```python
from build123d import *

# Parameters (mm, degrees)
SKETCH2_R           = 15.875
SKETCH2_R_2         = 2.54
BOSS_EXTRUDE1_DEPTH = 3.175
FILLET1_R           = 2.54


with BuildPart() as part:
    # Sketch2 → Boss-Extrude1 (new body)
    with BuildSketch(Plane.XY):
        Polygon((-508, 25.4), (-481.624580264, 25.4), (-457.99375, 25.4), (-431.8, 25.4), (-368.3, 25.4), (-368.3, -25.4), (-431.8, -25.4), (-457.99375, -25.4), (-481.624580264, -25.4), (-508, -25.4), align=None)
        with Locations((-469.9, 0)):
            Circle(SKETCH2_R, mode=Mode.SUBTRACT)
        with Locations((-495.3, 12.7)):
            Circle(SKETCH2_R_2, mode=Mode.SUBTRACT)
        with Locations((-495.3, -12.7)):
            Circle(SKETCH2_R_2, mode=Mode.SUBTRACT)
        with Locations((-444.5, -12.7)):
            Circle(SKETCH2_R_2, mode=Mode.SUBTRACT)
        with Locations((-431.8, -12.7)):
            Circle(SKETCH2_R_2, mode=Mode.SUBTRACT)
        with Locations((-419.1, -12.7)):
            Circle(SKETCH2_R_2, mode=Mode.SUBTRACT)
        with Locations((-419.1, 0)):
            Circle(SKETCH2_R_2, mode=Mode.SUBTRACT)
        with Locations((-431.8, 0)):
            Circle(SKETCH2_R_2, mode=Mode.SUBTRACT)
        with Locations((-431.8, 12.7)):
            Circle(SKETCH2_R_2, mode=Mode.SUBTRACT)
        with Locations((-419.1, 12.7)):
            Circle(SKETCH2_R_2, mode=Mode.SUBTRACT)
        with Locations((-444.5, 12.7)):
            Circle(SKETCH2_R_2, mode=Mode.SUBTRACT)
        with Locations((-406.4, 12.7)):
            Circle(SKETCH2_R_2, mode=Mode.SUBTRACT)
        with Locations((-406.4, 0)):
            Circle(SKETCH2_R_2, mode=Mode.SUBTRACT)
        with Locations((-406.4, -12.7)):
            Circle(SKETCH2_R_2, mode=Mode.SUBTRACT)
        with Locations((-393.7, 12.7)):
            Circle(SKETCH2_R_2, mode=Mode.SUBTRACT)
        with Locations((-393.7, 0)):
            Circle(SKETCH2_R_2, mode=Mode.SUBTRACT)
        with Locations((-393.7, -12.7)):
            Circle(SKETCH2_R_2, mode=Mode.SUBTRACT)
        with Locations((-381, 12.7)):
            Circle(SKETCH2_R_2, mode=Mode.SUBTRACT)
        with Locations((-381, 0)):
            Circle(SKETCH2_R_2, mode=Mode.SUBTRACT)
        with Locations((-381, -12.7)):
            Circle(SKETCH2_R_2, mode=Mode.SUBTRACT)
    extrude(amount=BOSS_EXTRUDE1_DEPTH)

    # Fillet1
    fillet1_edges = [part.edges().sort_by_distance(p)[0] for p in [
        (-508, 25.4, 1.5875),
        (-368.3, 25.4, 1.5875),
        (-368.3, -25.4, 1.5875),
        (-508, -25.4, 1.5875),
    ]]
    fillet(fillet1_edges, radius=FILLET1_R)


solid = part.part
```
Could you check a few things on this model? Use its own coordinates, in mm. Round coordinates to 2 decimals unless told otherwise and drop trailing zeros. Loops run counter-clockwise (first coordinate to the right, second up) from the corner with the lowest first, then second, coordinate; pieces in that order, holes last. Notation, with made-up numbers: (67, -25.75) - (122, -25.75) arc R20 cw to (122, 1.25) - close; hole circle Ø10 at (-5, 21). An arc over 180 degrees is marked (long way). Answer as CSV lines item,"result".
1. We'd pull the mould along Y, two halves only. Please class faces 1 (the face through (-369.024, -24.636, 1.61)), 2 (the face through (-416.754, -0.973, 1.565)), 3 (the face through (-437, 0, 3.175)): +Y half, -Y half, draft (parallel to the pull), parting line (faces both ways), or undercut.
Filled in:
face 1,"-Y half"
face 2,"undercut"
face 3,"draft"
2. Please list where these lines run through material, in increasing order: line 1 along Y through (x, z) = (-444.5, 1.75); line 2 along Y through (x, z) = (-381, 2); line 3 along Y through (x, z) = (-383, 3). Write a range as [from, to].
Filled in:
line 1,"y = [-25.4, -15.24], [-10.16, 10.16], [15.24, 25.4]"
line 2,"y = [-25.4, -15.24], [-10.16, -2.54], [2.54, 10.16], [15.24, 25.4]"
line 3,"y = [-25.4, -14.27], [-11.13, -1.57], [1.57, 11.13], [14.27, 25.4]"
3. I want a section at A-A on x = -469.9. List the corners of the cut face in (y, z) for me (3 decimals), then the cut area to 3 significant figures.
Filled in:
outline,"(-25.4, 0) - (-15.875, 0) - (-15.875, 3.175) - (-25.4, 3.175) - close; (15.875, 0) - (25.4, 0) - (25.4, 3.175) - (15.875, 3.175) - close"
area,"60.5 mm^2"
4. I want a section at B-B on y = 0. List the corners of the cut face in (x, z) for me (3 decimals), then the cut area to 3 significant figures.
Filled in:
outline,"(-508, 0) - (-485.775, 0) - (-485.775, 3.175) - (-508, 3.175) - close; (-454.025, 0) - (-434.34, 0) - (-434.34, 3.175) - (-454.025, 3.175) - close; (-429.26, 0) - (-421.64, 0) - (-421.64, 3.175) - (-429.26, 3.175) - close; (-416.56, 0) - (-408.94, 0) - (-408.94, 3.175) - (-416.56, 3.175) - close; (-403.86, 0) - (-396.24, 0) - (-396.24, 3.175) - (-403.86, 3.175) - close; (-391.16, 0) - (-383.54, 0) - (-383.54, 3.175) - (-391.16, 3.175) - close; (-378.46, 0) - (-368.3, 0) - (-368.3, 3.175) - (-378.46, 3.175) - close"
area,"262 mm^2"
5. I want a section at C-C on x = -419.1. List the corners of the cut face in (y, z) for me (3 decimals).
Filled in:
outline,"(-25.4, 0) - (-15.24, 0) - (-15.24, 3.175) - (-25.4, 3.175) - close; (-10.16, 0) - (-2.54, 0) - (-2.54, 3.175) - (-10.16, 3.175) - close; (2.54, 0) - (10.16, 0) - (10.16, 3.175) - (2.54, 3.175) - close; (15.24, 0) - (25.4, 0) - (25.4, 3.175) - (15.24, 3.175) - close"
6. I want a section at D-D on z = 1.3. Count the separate pieces of the cut face and the enclosed holes in it, then the cut area to 3 significant figures.
Filled in:
separate pieces,"1"
enclosed holes,"20"
area,"5,910 mm^2"
